Check sheet for the modelled part. Datum: model origin and axes. Units: mm. Coordinates: 2 decimals unless noted, no trailing zeros. Order: outer loops, then holes, each group sorted by start corner. A loop starts at its lowest first (then second) coordinate and runs counter-clockwise, first axis right, second up. Notation, with made-up numbers: (42, -26) -> (56, -26) arc R22 ccw to (56, 12) -> close; hole circle Ø8 at (-12, 40). An arc over 180 degrees is marked (long way). Put each result on its own line as item: value. Start each with the question number.
```python
from build123d import *

# Parameters (mm, degrees)
SKETCH1_W                                         = 38.1
SKETCH1_H                                         = 1.5875
CSK_FOR_0_FLAT_HEAD_MACHINE_SCREW_100_D           = 1.778
CSK_FOR_0_FLAT_HEAD_MACHINE_SCREW_100_CSINK_D     = 3.0226
CSK_FOR_0_FLAT_HEAD_MACHINE_SCREW_100_CSINK_ANGLE = 100
CIRPATTERN1_COUNT                                 = 12


with BuildPart() as part:
    # Sketch1 → Revolve1 (revolve)
    with BuildSketch(Plane.XY):
        with Locations((-25.4, 0.79375)):
            Rectangle(SKETCH1_W, SKETCH1_H)
    revolve(axis=Axis((0, 55, 0), (0, -1, 0)))

    # CSK for #0 Flat Head Machine Screw (100)1 (through all)
    with Locations(Plane(origin=(0, 1.5875, 0), x_dir=(1, 0, 0), z_dir=(0, 1, 0))):
        with Locations((-41.275, 0)):
            csk_for_0_flat_head_machine_screw_100 = CounterSinkHole(CSK_FOR_0_FLAT_HEAD_MACHINE_SCREW_100_D / 2, CSK_FOR_0_FLAT_HEAD_MACHINE_SCREW_100_CSINK_D / 2, counter_sink_angle=CSK_FOR_0_FLAT_HEAD_MACHINE_SCREW_100_CSINK_ANGLE)

    # CirPattern1: CSK for #0 Flat Head Machine Screw (100)1 ×12 about axis
    cirpattern1_axis = Axis((0, 0, 0), (0, 1, 0))
    for i in range(1, CIRPATTERN1_COUNT):
        add(csk_for_0_flat_head_machine_screw_100.rotate(cirpattern1_axis, i * 360 / CIRPATTERN1_COUNT), mode=Mode.SUBTRACT)


solid = part.part
```
1) Sectioned sample at A-A (x = -4). Record the boundary of the cut face in (y, z), plus the area to 3 significant figures.
2) Sectioned sample at D-D (x = -28). Record the boundary of the cut face in (y, z).
3) Gauge pin test, flat ends, axial feed: pin 1 (1.6 mm diameter, centred on x = 35.75, z = -20.64, fed in from -Y); pin 2 (2 mm diameter, centred on x = -20.64, z = 35.75, fed in from +Y); pin 3 (2 mm diameter, centred on x = -41.275, z = 0, fed in from -Y). Record the tip position at first contact, or that the pin passes through.
4) Scan lines: line 1 along Z through (x, y) = (-0.5, 1.05); line 2 along Z through (x, y) = (-14, 0.25); line 3 along Z through (x, y) = (3, 0.75). Record each from-to range of solid material in increasing order. Write a range as [from, to].
5) Mould release check, pull along X, two halves, no side actions. Record for faces 1 (the cylindrical face through (-2.93, 0.805, 5.634)), 2 (the flat face through (1, 1.587, 9)), 3 (the cylindrical face through (-42.397, 0.805, -13.352)): +X half, -X half, draft (parallel to the pull), parting line (faces both ways), or undercut.
6) Sectioned sample at B-B (y = 0.8). State how many separate pieces and enclosed holes the cut face has, plus the area to 3 significant figures.
7) Sectioned sample at C-C (z = 9). Record the boundary of the cut face in (x, y), plus the area to 3 significant figures.
Entries:
1. outline: (0, -44.27) -> (1.59, -44.27) -> (1.59, -4.93) -> (0, -4.93) -> close; (0, 4.93) -> (1.59, 4.93) -> (1.59, 44.27) -> (0, 44.27) -> close
1. area: 125 mm2
2. outline: (0, -34.52) -> (1.59, -34.52) -> (1.59, 34.52) -> (0, 34.52) -> close
3. pin 1: passes through
3. pin 2: stops at y = 1.16
3. pin 3: stops at y = 0
4. line 1: z = [-44.45, -42.01], [-40.54, -6.33], [6.33, 40.54], [42.01, 44.45]
4. line 2: z = [-42.19, 42.19]
4. line 3: z = [-44.35, -5.6], [5.6, 44.35]
5. face 1: undercut
5. face 2: draft
5. face 3: parting line
6. separate pieces: 1
6. enclosed holes: 13
6. area: 6,050 mm2
7. outline: (-43.53, 0) -> (43.53, 0) -> (43.53, 1.59) -> (-43.53, 1.59) -> close
7. area: 138 mm2
